CAD build for the part. Positions are in the model's coordinates, mm. A direction names the side the tool comes from. Round coordinates to 2 decimals unless told otherwise and drop trailing zeros. Loops run counter-clockwise (first coordinate to the right, second up) from the corner with the lowest first, then second, coordinate; pieces in that order, holes last. Notation, with made-up numbers: M 1,58 L 49,58 A8 cw 49,67 Z; hole C 21.5,-21.75 d7. An arc over 180 degrees is marked long. One line per item, written item: value. Start each with the question number.
from build123d import *

# Parameters (mm, degrees)
SKETCH1_W           = 52.084
SKETCH1_H           = 102.362
BOSS_EXTRUDE1_DEPTH = 6.35
SKETCH1_4_R         = 1.6
CUT_EXTRUDE2_DEPTH  = 116.026277867
SKETCH1_5_R         = 3.556
CUT_EXTRUDE3_DEPTH  = 4.7625
FILLET1_R           = 18
SKETCH1_7_W         = 17
SKETCH1_7_H         = 5
CUT_EXTRUDE4_DEPTH  = 116.026277867
FILLET4_R           = 3
SKETCH3_W           = 22.451753575
SKETCH3_H           = 92.950303638
CUT_EXTRUDE6_DEPTH  = 6.35


with BuildPart() as part:
    # Sketch1 → Boss-Extrude1 (new body)
    with BuildSketch(Plane(origin=(0, 0, 0), x_dir=(1, 0, 0), z_dir=(0, 1, 0))):
        with Locations((26.042, 51.181)):
            Rectangle(SKETCH1_W, SKETCH1_H)
    extrude(amount=BOSS_EXTRUDE1_DEPTH)

    # Sketch1<4> → Cut-Extrude2 (cut, through all)
    with BuildSketch(Plane(origin=(0, 0, 0), x_dir=(1, 0, 0), z_dir=(0, 1, 0))):
        with BuildLine():
            ThreePointArc((9.1, 71.772), (8.63137085, 72.90337085), (7.5, 73.372))
            Line((7.5, 73.372), (7.5, 70.172))
            ThreePointArc((7.5, 70.172), (8.63137085, 70.64062915), (9.1, 71.772))
        make_face()
        with BuildLine():
            Line((7.5, 70.172), (7.5, 73.372))
            ThreePointArc((7.5, 73.372), (5.9, 71.772), (7.5, 70.172))
        make_face()
        with Locations(Location((7.5, 92.362, 0), (0, 0, 270))):
            Circle(SKETCH1_4_R)
        with Locations(Location((7.5, 51.182, 0), (0, 0, 270))):
            Circle(SKETCH1_4_R)
        with Locations(Location((7.5, 30.592, 0), (0, 0, 270))):
            Circle(SKETCH1_4_R)
        with Locations(Location((7.5, 10.002, 0), (0, 0, 270))):
            Circle(SKETCH1_4_R)
    extrude(amount=CUT_EXTRUDE2_DEPTH, mode=Mode.SUBTRACT)

    # Sketch1<5> → Cut-Extrude3 (cut)
    with BuildSketch(Plane(origin=(0, 0, 0), x_dir=(1, 0, 0), z_dir=(0, 1, 0))):
        with Locations(Location((38.876, 95.63, 0), (0, 0, 90))):
            Circle(SKETCH1_5_R)
        with Locations(Location((38.876, 6.73, 0), (0, 0, 90))):
            Circle(SKETCH1_5_R)
        with BuildLine():
            Line((30.360375772, 43.18), (30.360375772, 59.18))
            ThreePointArc((30.360375772, 59.18), (50.56, 51.18), (30.360375772, 43.18))
        make_face()
    extrude(amount=CUT_EXTRUDE3_DEPTH, mode=Mode.SUBTRACT)

    # Fillet1
    fillet1_edges = [part.edges().sort_by_distance(p)[0] for p in [
        (52.084, 3.175, 0),
        (52.084, 3.175, -102.362),
    ]]
    fillet(fillet1_edges, radius=FILLET1_R)

    # Sketch1<7> → Cut-Extrude4 (cut, through all)
    with BuildSketch(Plane(origin=(0, 0, 0), x_dir=(1, 0, 0), z_dir=(0, 1, 0))):
        with Locations((8.5, 2.5)):
            Rectangle(SKETCH1_7_W, SKETCH1_7_H)
        with Locations((8.5, 99.862)):
            Rectangle(SKETCH1_7_W, SKETCH1_7_H)
    extrude(amount=CUT_EXTRUDE4_DEPTH, mode=Mode.SUBTRACT)

    # Fillet4
    fillet4_edges = [part.edges().sort_by_distance(p)[0] for p in [
        (0, 3.175, -5),
        (17, 3.175, 0),
        (0, 3.175, -97.362),
        (17, 3.175, -102.362),
    ]]
    fillet(fillet4_edges, radius=FILLET4_R)

    # Sketch3 → Cut-Extrude6 (cut)
    with BuildSketch(Plane.XZ):
        with Locations((57.445177666, -51.181)):
            Rectangle(SKETCH3_W, SKETCH3_H)
    extrude(amount=-CUT_EXTRUDE6_DEPTH, mode=Mode.SUBTRACT)


solid = part.part
(1) Slice it at C-C, the plane x = 32.5. List the corners of the cut face in (y, z).
(2) Flat gauge pins, fed straight in: P1, Ø0.6, axis at y = 2.5, z = -3.5, coming from the -X side; P2, Ø17.5, axis at x = 40.5, z = -49.5, coming from the -Y side; P3, Ø1.5, axis at y = 2.5, z = -49, coming from the +X side; P4, Ø5.5, axis at x = 40.5, z = -94, coming from the -Y side. Where does each tip first touch, or does it go through?
(3) Which spindle directions (+Z, -Z, +X, -X, +Y, -Y) get a long thin tool onto all of the face, cutting with end or side? Do faces 1 (the flat face through (30.36, 2, -51)), 2 (the flat face through (39, 4.762, -96)), 3 (the flat face through (10, 3, -5)). Say none if no direction does.
(4) Slice it at B-B, the plane z = -95.63. List the corners of the cut face in (x, y).
(5) Mould opens along Z. For faces 4 (the cylindrical face through (7.981, 3.131, -90.836)), 5 (the cylindrical face through (17.9, 3.22, -0.86)), 6 (the cylindrical face through (40.5, 3.22, -101.18)) say: pulls with the +Z half, pulls with the -Z half, needs draft (parallel to the pull), parting line crosses it, or undercut.
(6) Slice it at A-A, the plane y = 3.25. List the corners of the cut face in (x, z), and give its area (3 significant figures).
(7) Probe L1, parallel to Z at x = 7.5, y = 3.25; L2, parallel to Z at x = 36, y = 2; L3, parallel to Z at x = 16, y = 1. List the from-to ranges inside material, lowest first.
Check result:
1. outline: M 0,-102.36 L 6.35,-102.36 L 6.35,0 L 0,0 L 0,-41.39 L 4.76,-41.39 L 4.76,-60.97 L 0,-60.97 Z
2. P1: stops at x = 17
2. P2: stops at y = 4.76
2. P3: stops at x = 30.36
2. P4: stops at y = 0
3. face 1: +X, -Y
3. face 2: -Y
3. face 3: +Z, -X, +Y, -Y
4. outline: M 0.28,0 L 35.32,0 L 35.32,4.76 L 42.43,4.76 L 42.43,0 L 46.22,0 L 46.22,6.35 L 0.28,6.35 Z
5. face 4: undercut
5. face 5: pulls with the +Z half
5. face 6: pulls with the -Z half
6. outline: M 0,-94.36 A3 ccw 3,-97.36 L 17,-97.36 L 17,-99.36 A3 ccw 20,-102.36 L 34.08,-102.36 A18 ccw 46.22,-97.66 L 46.22,-60.27 A11.68 cw 30.36,-59.18 L 30.36,-43.18 A11.68 cw 46.22,-42.09 L 46.22,-4.71 A18 ccw 34.08,0 L 20,0 A3 ccw 17,-3 L 17,-5 L 3,-5 A3 ccw 0,-8 Z; hole C 7.5,-92.36 d3.2; hole C 7.5,-71.77 d3.2; hole C 7.5,-51.18 d3.2; hole C 7.5,-30.59 d3.2; hole C 7.5,-10 d3.2; hole C 38.88,-95.63 d7.11; hole C 38.88,-6.73 d7.11
6. area: 4,060 mm^2
7. L1: z = -97.36 to -93.96, -90.76 to -73.37, -70.17 to -52.78, -49.58 to -32.19, -28.99 to -11.6, -8.4 to -5
7. L2: z = -102.26 to -97.72, -93.54 to -62.5, -39.86 to -8.82, -4.64 to -0.1
7. L3: z = -97.36 to -5
